Can you work these out from the model? Positions are in its coordinate system, mm. A direction names the side the tool comes from. Give positions to 0.01 mm unless a question says otherwise; leave off trailing zeros. One line per question, with ' | ' between items. Start each with the question number.
1) Thinking about a two-plate mould opening in Y: for faces 4 (the flat face through (0, 3, 203.225)), 5 (the flat face through (-5.41, -6.92, 100.19)), 6 (the flat face through (0, 4.382, 103)), which applies, +Y half, -Y half, draft (parallel to the pull), parting line (faces both ways), or undercut?
2) I'm going to push flat-ended pins straight in: pin 1 Ø12 at (x, z) = (4, 162) entering from +Y; pin 2 Ø0.7 at (y, z) = (-6, 65) entering from -X; pin 3 Ø4 at (x, z) = (10, 145.5) entering from -Y. Where does each tip first touch, or does it pass through?
3) For faces 1 (the flat face through (-4.382, 0, 103)), 2 (the flat face through (4.382, 0, 103)), 3 (the flat face through (-6.88, -5.37, 100.19)), which set-ups out of +Z, -Z, +X, -X, +Y, -Y let a thin tool reach every point of the face, with its end or its side?
4) Please list where these lines run through material, in increasing order: line 1 along X through (y, z) = (6.5, 139); line 2 along Y through (x, z) = (0, 120); line 3 along Y through (x, z) = (6, 57.5). Write a range as [from, to].
```python
from build123d import *

# Parameters (mm, degrees)
BOSS_EXTRUDE1_DEPTH   = 203.2254
BOSS_EXTRUDE1_2_DEPTH = 203.2254
BOSS_EXTRUDE1_3_DEPTH = 203.2254
BOSS_EXTRUDE1_4_DEPTH = 203.2254
FILLET1_R             = 1.0922
FILLET2_R             = 1.0922
FILLET3_R             = 1.016
FILLET4_R             = 1.016
FILLET5_R             = 0.254
FILLET6_R             = 0.254
FILLET7_R             = 0.254
FILLET8_R             = 0.254
FILLET9_R             = 1.016
FILLET10_R            = 1.0922
FILLET11_R            = 1.0922
FILLET12_R            = 1.0922
FILLET13_R            = 1.0922
FILLET14_R            = 1.0922
SKETCH2_W             = 8.763
SKETCH2_H             = 8.763
SKETCH2_R             = 2.5019
BOSS_EXTRUDE2_DEPTH   = 203.2254
FILLET15_R            = 3.175


with BuildPart() as part:
    # Sketch1 → Boss-Extrude1 (new body)
    with BuildSketch(Plane.XY):
        Polygon((-8.714816972, 10.2235), (-4.3815, 10.2235), (-4.3815, 12.225663986), (-12.5095, 12.5095), (-12.225663986, 4.3815), (-10.2235, 4.3815), (-10.2235, 8.714816972), (-4.3815, 2.872816972), (-4.3815, 4.3815), (-2.872816972, 4.3815), align=None)
    extrude(amount=BOSS_EXTRUDE1_DEPTH)

    # Fillet1
    # the kernel refuses this fillet: 1.0922 mm, written as the material it takes off along each edge
    with BuildSketch(Plane(origin=(-4.3815, 10.2235, -2.7305), x_dir=(-1, 0, 0), z_dir=(0, 0, 1))) as fillet1_piece_1:
        with BuildLine():
            CenterArc((FILLET1_R, -FILLET1_R), FILLET1_R, 90, 90)
            Line((0, -FILLET1_R), (0, 0))
            Line((0, 0), (FILLET1_R, 0))
        make_face()
    extrude(amount=208.6864, mode=Mode.SUBTRACT)
    with BuildSketch(Plane(origin=(-4.3815, 12.225663986, -2.6368132), x_dir=(0, -1, 0), z_dir=(0, 0, 1))) as fillet1_piece_2:
        with BuildLine():
            CenterArc((FILLET1_R * 0.965688774807, -FILLET1_R), FILLET1_R, 90, 88)
            Line((-FILLET1_R * 0.033702052212, -FILLET1_R * 0.965100503298), (0, 0))
            Line((0, 0), (FILLET1_R * 0.965688774807, 0))
        make_face()
    extrude(amount=208.499026399, mode=Mode.SUBTRACT)

    # Fillet2
    # the kernel refuses this fillet: 1.0922 mm, written as the material it takes off along each edge
    with BuildSketch(Plane(origin=(-10.2235, 4.3815, -2.7305), x_dir=(0, 1, 0), z_dir=(0, 0, 1))) as fillet2_piece_1:
        with BuildLine():
            CenterArc((FILLET2_R, FILLET2_R), FILLET2_R, 180, 90)
            Line((0, FILLET2_R), (0, 0))
            Line((0, 0), (FILLET2_R, 0))
        make_face()
    extrude(amount=208.6864, mode=Mode.SUBTRACT)
    with BuildSketch(Plane(origin=(-12.225663986, 4.3815, -2.6368132), x_dir=(1, 0, 0), z_dir=(0, 0, 1))) as fillet2_piece_2:
        with BuildLine():
            CenterArc((FILLET2_R * 0.965688774807, FILLET2_R), FILLET2_R, 182, 88)
            Line((-FILLET2_R * 0.033702052212, FILLET2_R * 0.965100503298), (0, 0))
            Line((0, 0), (FILLET2_R * 0.965688774807, 0))
        make_face()
    extrude(amount=208.499026399, mode=Mode.SUBTRACT)

    # Fillet3
    fillet3_edges = [part.edges().sort_by_distance(p)[0] for p in [
        (-10.2235, 8.714816972, 101.6127),
    ]]
    fillet(fillet3_edges, radius=FILLET3_R)

    # Fillet4
    fillet4_edges = [part.edges().sort_by_distance(p)[0] for p in [
        (-8.714816972, 10.2235, 101.6127),
    ]]
    fillet(fillet4_edges, radius=FILLET4_R)

    # Fillet5
    fillet5_edges = [part.edges().sort_by_distance(p)[0] for p in [
        (-12.5095, 12.5095, 101.6127),
    ]]
    fillet(fillet5_edges, radius=FILLET5_R)



with BuildPart() as body_2:
    # Sketch1 → Boss-Extrude1 2 (new body)
    with BuildSketch(Plane.XY):
        Polygon((12.5095, 12.5095), (4.3815, 12.225663986), (4.3815, 10.2235), (8.714816972, 10.2235), (2.872816972, 4.3815), (4.3815, 4.3815), (4.3815, 2.872816972), (10.2235, 8.714816972), (10.2235, 4.3815), (12.225663986, 4.3815), align=None)
    extrude(amount=BOSS_EXTRUDE1_2_DEPTH)

    # Fillet7
    fillet7_edges = [body_2.edges().sort_by_distance(p)[0] for p in [
        (12.5095, 12.5095, 101.6127),
    ]]
    fillet(fillet7_edges, radius=FILLET7_R)

    # Fillet11
    # the kernel refuses this fillet: 1.0922 mm, written as the material it takes off along each edge
    with BuildSketch(Plane(origin=(4.3815, 10.2235, -2.7305), x_dir=(0, 1, 0), z_dir=(0, 0, 1))) as fillet11_piece_1:
        with BuildLine():
            CenterArc((FILLET11_R, -FILLET11_R), FILLET11_R, 90, 90)
            Line((0, -FILLET11_R), (0, 0))
            Line((0, 0), (FILLET11_R, 0))
        make_face()
    extrude(amount=208.6864, mode=Mode.SUBTRACT)
    with BuildSketch(Plane(origin=(4.3815, 12.225663986, -2.6368132), x_dir=(0.9993908270190961, 0.03489949670249208, 0), z_dir=(0, 0, 1))) as fillet11_piece_2:
        with BuildLine():
            CenterArc((FILLET11_R * 0.965688774807, -FILLET11_R), FILLET11_R, 90, 88)
            Line((-FILLET11_R * 0.033702052212, -FILLET11_R * 0.965100503298), (0, 0))
            Line((0, 0), (FILLET11_R * 0.965688774807, 0))
        make_face()
    extrude(amount=208.499026399, mode=Mode.SUBTRACT)
    with BuildSketch(Plane(origin=(10.2235, 4.3815, -2.7305), x_dir=(1, 0, 0), z_dir=(0, 0, 1))) as fillet11_piece_3:
        with BuildLine():
            CenterArc((FILLET11_R, FILLET11_R), FILLET11_R, 180, 90)
            Line((0, FILLET11_R), (0, 0))
            Line((0, 0), (FILLET11_R, 0))
        make_face()
    extrude(amount=208.6864, mode=Mode.SUBTRACT)
    with BuildSketch(Plane(origin=(12.225663986, 4.3815, -2.6368132), x_dir=(0.03489949670249721, 0.9993908270190958, 0), z_dir=(0, 0, 1))) as fillet11_piece_4:
        with BuildLine():
            CenterArc((FILLET11_R * 0.965688774807, FILLET11_R), FILLET11_R, 182, 88)
            Line((-FILLET11_R * 0.033702052212, FILLET11_R * 0.965100503298), (0, 0))
            Line((0, 0), (FILLET11_R * 0.965688774807, 0))
        make_face()
    extrude(amount=208.499026399, mode=Mode.SUBTRACT)

    # Fillet14
    fillet14_edges = [body_2.edges().sort_by_distance(p)[0] for p in [
        (10.2235, 8.714816972, 101.6127),
        (8.714816972, 10.2235, 101.6127),
    ]]
    fillet(fillet14_edges, radius=FILLET14_R)


with BuildPart() as body_3:
    # Sketch1 → Boss-Extrude1 3 (new body)
    with BuildSketch(Plane.XY):
        Polygon((12.5095, -12.5095), (12.225663986, -4.3815), (10.2235, -4.3815), (10.2235, -8.714816972), (4.3815, -2.872816972), (4.3815, -4.3815), (2.872816972, -4.3815), (8.714816972, -10.2235), (4.3815, -10.2235), (4.3815, -12.225663986), align=None)
    extrude(amount=BOSS_EXTRUDE1_3_DEPTH)

    # Fillet8
    fillet8_edges = [body_3.edges().sort_by_distance(p)[0] for p in [
        (12.5095, -12.5095, 101.6127),
    ]]
    fillet(fillet8_edges, radius=FILLET8_R)

    # Fillet12
    # the kernel refuses this fillet: 1.0922 mm, written as the material it takes off along each edge
    with BuildSketch(Plane(origin=(12.225663986, -4.3815, -2.6368132), x_dir=(0.03489949670249375, -0.999390827019096, 0), z_dir=(0, 0, 1))) as fillet12_piece_1:
        with BuildLine():
            CenterArc((FILLET12_R * 0.965688774807, -FILLET12_R), FILLET12_R, 90, 88)
            Line((-FILLET12_R * 0.033702052212, -FILLET12_R * 0.965100503298), (0, 0))
            Line((0, 0), (FILLET12_R * 0.965688774807, 0))
        make_face()
    extrude(amount=208.499026399, mode=Mode.SUBTRACT)
    with BuildSketch(Plane(origin=(10.2235, -4.3815, -2.7305), x_dir=(1, 0, 0), z_dir=(0, 0, 1))) as fillet12_piece_2:
        with BuildLine():
            CenterArc((FILLET12_R, -FILLET12_R), FILLET12_R, 90, 90)
            Line((0, -FILLET12_R), (0, 0))
            Line((0, 0), (FILLET12_R, 0))
        make_face()
    extrude(amount=208.6864, mode=Mode.SUBTRACT)
    with BuildSketch(Plane(origin=(4.3815, -12.225663986, -2.6368132), x_dir=(0.9993908270190958, -0.03489949670249721, 0), z_dir=(0, 0, 1))) as fillet12_piece_3:
        with BuildLine():
            CenterArc((FILLET12_R * 0.965688774807, FILLET12_R), FILLET12_R, 182, 88)
            Line((-FILLET12_R * 0.033702052212, FILLET12_R * 0.965100503298), (0, 0))
            Line((0, 0), (FILLET12_R * 0.965688774807, 0))
        make_face()
    extrude(amount=208.499026399, mode=Mode.SUBTRACT)
    with BuildSketch(Plane(origin=(4.3815, -10.2235, -2.7305), x_dir=(0, -1, 0), z_dir=(0, 0, 1))) as fillet12_piece_4:
        with BuildLine():
            CenterArc((FILLET12_R, FILLET12_R), FILLET12_R, 180, 90)
            Line((0, FILLET12_R), (0, 0))
            Line((0, 0), (FILLET12_R, 0))
        make_face()
    extrude(amount=208.6864, mode=Mode.SUBTRACT)

    # Fillet13
    fillet13_edges = [body_3.edges().sort_by_distance(p)[0] for p in [
        (8.714816972, -10.2235, 101.6127),
        (10.2235, -8.714816972, 101.6127),
    ]]
    fillet(fillet13_edges, radius=FILLET13_R)


with BuildPart() as body_4:
    # Sketch1 → Boss-Extrude1 4 (new body)
    with BuildSketch(Plane.XY):
        Polygon((-12.5095, -12.5095), (-4.3815, -12.225663986), (-4.3815, -10.2235), (-8.714816972, -10.2235), (-2.872816972, -4.3815), (-4.3815, -4.3815), (-4.3815, -2.872816972), (-10.2235, -8.714816972), (-10.2235, -4.3815), (-12.225663986, -4.3815), align=None)
    extrude(amount=BOSS_EXTRUDE1_4_DEPTH)

    # Fillet6
    fillet6_edges = [body_4.edges().sort_by_distance(p)[0] for p in [
        (-12.5095, -12.5095, 101.6127),
    ]]
    fillet(fillet6_edges, radius=FILLET6_R)

    # Fillet9
    fillet9_edges = [body_4.edges().sort_by_distance(p)[0] for p in [
        (-10.2235, -8.714816972, 101.6127),
        (-8.714816972, -10.2235, 101.6127),
    ]]
    fillet(fillet9_edges, radius=FILLET9_R)

    # Fillet10
    # the kernel refuses this fillet: 1.0922 mm, written as the material it takes off along each edge
    with BuildSketch(Plane(origin=(-4.3815, -10.2235, -2.7305), x_dir=(-1, 0, 0), z_dir=(0, 0, 1)), Plane(origin=(-10.2235, -4.3815, -2.7305), x_dir=(-1, 0, 0), z_dir=(0, 0, 1))) as fillet10_piece_1:
        with BuildLine():
            CenterArc((FILLET10_R, FILLET10_R), FILLET10_R, 180, 90)
            Line((0, FILLET10_R), (0, 0))
            Line((0, 0), (FILLET10_R, 0))
        make_face()
    extrude(amount=208.6864, mode=Mode.SUBTRACT)
    with BuildSketch(Plane(origin=(-4.3815, -12.225663986, -2.6368132), x_dir=(0, 1, 0), z_dir=(0, 0, 1)), Plane(origin=(-12.225663986, -4.3815, -2.6368132), x_dir=(-0.03489949670249721, -0.9993908270190958, 0), z_dir=(0, 0, 1))) as fillet10_piece_2:
        with BuildLine():
            CenterArc((FILLET10_R * 0.965688774807, FILLET10_R), FILLET10_R, 182, 88)
            Line((-FILLET10_R * 0.033702052212, FILLET10_R * 0.965100503298), (0, 0))
            Line((0, 0), (FILLET10_R * 0.965688774807, 0))
        make_face()
    extrude(amount=208.499026399, mode=Mode.SUBTRACT)


with BuildPart() as part_1:
    add(part.part)

    add(body_2.part)  # Boss-Extrude2 merges body 2

    add(body_3.part)  # Boss-Extrude2 merges body 3

    add(body_4.part)  # Boss-Extrude2 merges body 4
    # Sketch2 → Boss-Extrude2 (add)
    with BuildSketch(Plane.XY.offset(203.2254)):
        Rectangle(SKETCH2_W, SKETCH2_H)
        Circle(SKETCH2_R, mode=Mode.SUBTRACT)
    extrude(amount=-BOSS_EXTRUDE2_DEPTH)

    # Fillet15
    fillet15_edges = [part_1.edges().sort_by_distance(p)[0] for p in [
        (4.3815, -2.872816972, 101.6127),
        (2.872816972, -4.3815, 101.6127),
        (-2.872816972, -4.3815, 101.6127),
        (-4.3815, -2.872816972, 101.6127),
        (-2.872816972, 4.3815, 101.6127),
        (-4.3815, 2.872816972, 101.6127),
        (2.872816972, 4.3815, 101.6127),
        (4.3815, 2.872816972, 101.6127),
    ]]
    fillet(fillet15_edges, radius=FILLET15_R)


solid = part_1.part
```
Results found:
1) face 4: draft | face 5: undercut | face 6: +Y half
2) pin 1: stops at y = 12.42 | pin 2: stops at x = -12.29 | pin 3: stops at y = -12.49
3) face 1: +Z, -Z, -X | face 2: +Z, -Z, +X | face 3: +Z, -Z
4) line 1: x = [-12.3, -10.2], [-8.01, -4.99], [4.99, 8.01], [10.14, 12.3] | line 2: y = [-4.38, -2.5], [2.5, 4.38] | line 3: y = [-12.28, -10.22], [-7.51, -4.49], [4.49, 7.51], [10.22, 12.28]
